```python
from build123d import *

# Parameters (mm, degrees)
SCHIZZO1_R                   = 235
ESTRUSIONE_ESTRUSIONE1_DEPTH = 20
SCHIZZO2_R                   = 235
SCHIZZO2_R_2                 = 225
ESTRUSIONE_ESTRUSIONE2_DEPTH = 10
SCHIZZO3_W                   = 30
SCHIZZO3_H                   = 30
ESTRUSIONE_ESTRUSIONE3_DEPTH = 30


with BuildPart() as part:
    # Schizzo1 → Estrusione-Estrusione1 (new body)
    with BuildSketch(Plane.XY):
        Circle(SCHIZZO1_R)
    extrude(amount=ESTRUSIONE_ESTRUSIONE1_DEPTH)

    # Schizzo2 → Estrusione-Estrusione2 (add)
    with BuildSketch(Plane.XY.offset(20)):
        Circle(SCHIZZO2_R)
        Circle(SCHIZZO2_R_2, mode=Mode.SUBTRACT)
    extrude(amount=ESTRUSIONE_ESTRUSIONE2_DEPTH)

    # Schizzo3 → Estrusione-Estrusione3 (add)
    with BuildSketch(Plane.XY.offset(20)):
        Rectangle(SCHIZZO3_W, SCHIZZO3_H)
    extrude(amount=ESTRUSIONE_ESTRUSIONE3_DEPTH)


solid = part.part
```
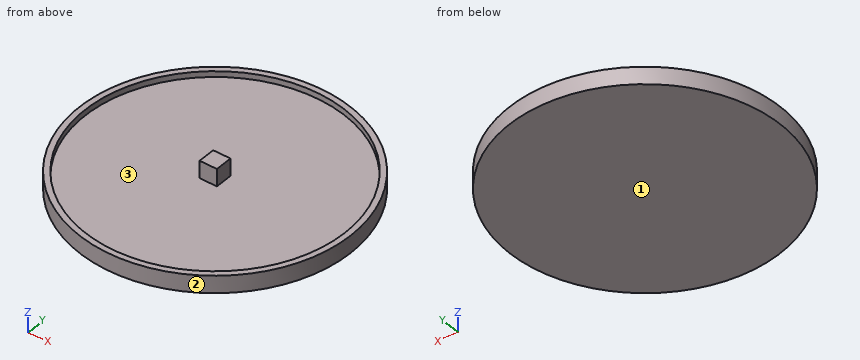
Design review of the part built by this model. Coordinates are the model's own, in mm. Face numbers are marked on the shaded views. Coordinates: 2 decimals unless noted, no trailing zeros. Order: outer loops, then holes, each group sorted by start corner. A loop starts at its lowest first (then second) coordinate and runs counter-clockwise, first axis right, second up.
1) Mouldability with a two-part tool opening along X and no side actions: class the marked faces 1, 2 and 3 as +X half, -X half, draft (parallel to the pull), parting line (faces both ways), or undercut.
2) Take a section at C-C, the plane z = 12. Give the boundary of the cut face in (x, y).
3) Take a section at D-D, the plane y = 102. Give the boundary of the cut face in (x, z), and give its area (3 significant figures).
4) Clearance check with flat-ended pins moving along their axes: pin 1 (5 mm diameter, centred on x = 150, z = 22, fed in from +Y); pin 2 (1.5 mm diameter, centred on x = -13.5, z = 37.5, fed in from -Y); pin 3 (1.5 mm diameter, centred on x = -36.5, z = 11.5, fed in from -Y). State where each tip first meets the part, or that it passes through.
5) Take a section at A-A, the plane y = 0. Give the boundary of the cut face in (x, z).
6) Wall thickness on line 1 along Y through (x, z) = (0, 23.5); line 2 along X through (y, z) = (-13.5, 25.5); line 3 along Z through (x, y) = (-34.5, -62): over which ranges is each line inside the solid? List them lowest first.
Returned:
1. face 1: draft
1. face 2: parting line
1. face 3: undercut
2. outline: circle Ø470 at (0, 0)
3. outline: (-211.71, 0) - (211.71, 0) - (211.71, 30) - (200.55, 30) - (200.55, 20) - (-200.55, 20) - (-200.55, 30) - (-211.71, 30) - close
3. area: 8,690 mm2
4. pin 1: stops at y = 182.94
4. pin 2: stops at y = -15
4. pin 3: stops at y = -232.26
5. outline: (-235, 0) - (235, 0) - (235, 30) - (225, 30) - (225, 20) - (15, 20) - (15, 50) - (-15, 50) - (-15, 20) - (-225, 20) - (-225, 30) - (-235, 30) - close
6. line 1: y = -235 to -225, -15 to 15, 225 to 235
6. line 2: x = -234.61 to -224.59, -15 to 15, 224.59 to 234.61
6. line 3: z = 0 to 20
